from build123d import *

# Parameters (mm, degrees)
SKETCH_1_W          = 183
SKETCH_1_H          = 179
EXTRUDE_1_DEPTH     = 36
CUT_EXTRUDE_1_DEPTH = 3
SKETCH_3_R          = 3
SKETCH_3_W          = 10
SKETCH_3_H          = 5
SKETCH_3_W_2        = 13.5
SKETCH_3_H_2        = 6
CUT_EXTRUDE_2_DEPTH = 10
SKETCH_4_R          = 6.5
EXTRUDE_2_DEPTH     = 1
SKETCH_5_R          = 2.5
SKETCH_5_W          = 17
SKETCH_5_H          = 6
SKETCH_5_W_2        = 13
SKETCH_5_W_3        = 15
SKETCH_5_H_2        = 11
CUT_EXTRUDE_3_DEPTH = 10
SKETCH_6_R          = 5
EXTRUDE_3_DEPTH     = 7.5


with BuildPart() as part:
    # 草图1 → 凸台-拉伸1 (new body)
    with BuildSketch(Plane(origin=(0, 0, 0), x_dir=(1, 0, 0), z_dir=(0, 1, 0))):
        Rectangle(SKETCH_1_W, SKETCH_1_H)
    extrude(amount=EXTRUDE_1_DEPTH)

    # 草图2 → 切除-拉伸1 (cut)
    with BuildSketch(Plane.XY.offset(89.5)):
        Polygon((-91.5, 36), (-91.5, 23), (30.5, 23), (30.5, 0), (91.5, 0), (91.5, 36), align=None)
    extrude(amount=-CUT_EXTRUDE_1_DEPTH, mode=Mode.SUBTRACT)

    # 草图3 → 切除-拉伸2 (cut)
    with BuildSketch(Plane.XY.offset(89.5)):
        with Locations((-56, 11)):
            Circle(SKETCH_3_R)
        with Locations((-45.5, 11)):
            Circle(SKETCH_3_R)
        with Locations((-27.5, 10.5)):
            Rectangle(SKETCH_3_W, SKETCH_3_H)
        with Locations((-7.25, 11)):
            Rectangle(SKETCH_3_W_2, SKETCH_3_H_2)
    extrude(amount=-CUT_EXTRUDE_2_DEPTH, mode=Mode.SUBTRACT)

    # 草图4 → 凸台-拉伸2 (add)
    with BuildSketch(Plane.XY.offset(89.5)):
        with Locations((-81.5, 11)):
            Circle(SKETCH_4_R)
    extrude(amount=EXTRUDE_2_DEPTH)

    # 草图5 → 切除-拉伸3 (cut)
    with BuildSketch(Plane(origin=(0, 0, -89.5), x_dir=(-1, 0, 0), z_dir=(0, 0, -1))):
        with Locations((-78, 11)):
            Circle(SKETCH_5_R)
        with Locations((-60, 11)):
            Rectangle(SKETCH_5_W, SKETCH_5_H)
        with Locations((-37, 11)):
            Rectangle(SKETCH_5_W, SKETCH_5_H)
        with Locations((16, 19.5)):
            Rectangle(SKETCH_5_W_2, SKETCH_5_H)
        with Locations((35, 19.5)):
            Rectangle(SKETCH_5_W_2, SKETCH_5_H)
        with Locations((16, 11)):
            Rectangle(SKETCH_5_W_2, SKETCH_5_H)
        with Locations((35, 11)):
            Rectangle(SKETCH_5_W_2, SKETCH_5_H)
        with Locations((59, 9.5)):
            Rectangle(SKETCH_5_W_3, SKETCH_5_H_2)
    extrude(amount=-CUT_EXTRUDE_3_DEPTH, mode=Mode.SUBTRACT)

    # 草图6 → 凸台-拉伸3 (add)
    with BuildSketch(Plane(origin=(0, 0, -89.5), x_dir=(-1, 0, 0), z_dir=(0, 0, -1))):
        with Locations((82.5, 24)):
            Circle(SKETCH_6_R)
    extrude(amount=EXTRUDE_3_DEPTH)


solid = part.part
Design review of the part built by this model. Coordinates are the model's own, in mm. A direction names the side the tool comes from. Coordinates: 2 decimals unless noted, no trailing zeros. Loops run counter-clockwise (first coordinate to the right, second up) from the corner with the lowest first, then second, coordinate; pieces in that order, holes last. Notation, with made-up numbers: (-19, 29.25) -> (37, 29.25) arc R21 cw to (37, 46.25) -> close; hole circle Ø11 at (-29.75, -21.5). An arc over 180 degrees is marked (long way). Use a Markdown table: item, result. Add a question column.
Item 1: Wall thickness on L1, parallel to Z at x = 77.5, y = 31; L2, parallel to Z at x = 1.5, y = 11.5: over which ranges is each line inside the solid? List them lowest first. Write a range as from..to.
Item 2: The part is to be moulded in two halves that separate along Y. For faces 1 (the flat face through (-1, 36, -3)), 2 (the flat face through (-59, 10, -79.5)), 3 (the flat face through (19, 26, 86.5)), 4 (the flat face through (-0.5, 11, 85)), say which applies: +Y half, -Y half, draft (parallel to the pull), parting line (faces both ways), or undercut.
Item 3: Machinability: for faces 5 (the flat face through (-91.5, 18, 1)), 6 (the flat face through (-56, 11, 79.5)), 7 (the flat face through (-66.5, 9, -85)), which of the approach directions +Z, -Z, +X, -X, +Y, -Y give a long, thin tool a straight path to every point of the face, cutting with its end or side? Answer none if there is none.
Item 4: We need section C-C, the plane x = 35. Write out the cut boundary in (y, z).
Item 5: Clearance check with flat-ended pins moving along their axes: P1, Ø6.5, axis at x = 33.5, y = 10.5, coming from the -Z side; P2, Ø5.5, axis at x = -57.5, y = 10, coming from the -Z side; P3, Ø9.5, axis at x = -56, y = 11, coming from the +Z side. State where each tip first meets the part, or that it passes through.
Item 6: We need section A-A, the plane x = -45.5. Write out the cut boundary in (y, z).
Item 7: We need section B-B, the plane y = 26.5. Write out the cut boundary in (x, z), and give its area (3 significant figures).
Numbers:
| question | item | result |
|---|---|---|
| 1 | L1 | z = -89.5..86.5 |
| 1 | L2 | z = -89.5..89.5 |
| 2 | face 1 | +Y half |
| 2 | face 2 | undercut |
| 2 | face 3 | draft |
| 2 | face 4 | undercut |
| 3 | face 5 | +Z, -Z, -X, +Y, -Y |
| 3 | face 6 | +Z |
| 3 | face 7 | -Z |
| 4 | outline | (0, -89.5) -> (8, -89.5) -> (8, -79.5) -> (14, -79.5) -> (14, -89.5) -> (36, -89.5) -> (36, 86.5) -> (0, 86.5) -> close |
| 5 | P1 | stops at z = -89.5 |
| 5 | P2 | stops at z = -79.5 |
| 5 | P3 | stops at z = 89.5 |
| 6 | outline | (0, -89.5) -> (36, -89.5) -> (36, 86.5) -> (23, 86.5) -> (23, 89.5) -> (14, 89.5) -> (14, 79.5) -> (8, 79.5) -> (8, 89.5) -> (0, 89.5) -> close |
| 7 | outline | (-91.5, -89.5) -> (-86.83, -89.5) -> (-86.83, -97) -> (-78.17, -97) -> (-78.17, -89.5) -> (91.5, -89.5) -> (91.5, 86.5) -> (-91.5, 86.5) -> close |
| 7 | area | 32,300 mm^2 |
